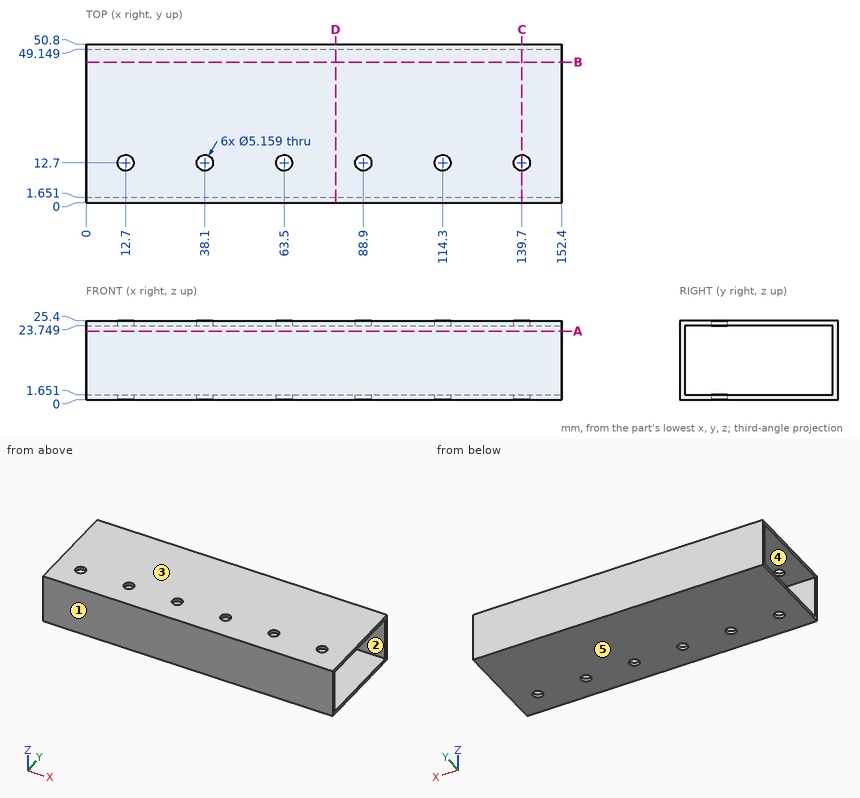
The drawing under review shows one solid part. Ordinate dimensions are in mm from its lowest x, y, z. A direction names the side the tool comes from. Coordinates: 2 decimals unless noted, no trailing zeros. Write each loop counter-clockwise with the first axis right and the second up, starting at its lowest first coordinate (ties: lowest second). Pieces come first, ordered by that corner, then holes. Notation, with made-up numbers: (6.5, 67) - (30.5, 67) arc R21 ccw to (30.5, 80) - close; hole circle Ø7 at (15, 33.25). An arc over 180 degrees is marked (long way). Use one line per item in the form item = value.
Q1. Consider section D-D (x = 80). Write out the cut boundary in (y, z).
Taken from the geometry:
outline = (0, 0) - (50.8, 0) - (50.8, 25.4) - (0, 25.4) - close; hole (1.65, 1.65) - (49.15, 1.65) - (49.15, 23.75) - (1.65, 23.75) - close
Q2. Consider section C-C (x = 139.7). Write out the cut boundary in (y, z).
Taken from the geometry:
outline = (0, 0) - (10.12, 0) - (10.12, 1.65) - (1.65, 1.65) - (1.65, 23.75) - (10.12, 23.75) - (10.12, 25.4) - (0, 25.4) - close; (15.28, 0) - (50.8, 0) - (50.8, 25.4) - (15.28, 25.4) - (15.28, 23.75) - (49.15, 23.75) - (49.15, 1.65) - (15.28, 1.65) - close
Q3. The part is to be moulded in two halves that separate along Z. For the marked faces 3, 4 and 5, say which applies: +Z half, -Z half, draft (parallel to the pull), parting line (faces both ways), or undercut.
Taken from the geometry:
face_3 = +Z half
face_4 = undercut
face_5 = -Z half
Q4. Machinability: for the marked faces 1 and 2, which of the approach directions +Z, -Z, +X, -X, +Y, -Y give a long, thin tool a straight path to every point of the face, cutting with its end or side? Answer none if there is none.
Taken from the geometry:
face_1 = +Z, -Z, +X, -X, -Y
face_2 = +X, -X
Q5. Consider section B-B (y = 45). Write out the cut boundary in (x, z).
Taken from the geometry:
outline = (0, 0) - (152.4, 0) - (152.4, 1.65) - (0, 1.65) - close; (0, 23.75) - (152.4, 23.75) - (152.4, 25.4) - (0, 25.4) - close
Q6. For probe 1 along Z at (x, y) = (99.5, 6.5); probe 2 along Y at (x, z) = (12.7, 0.9); probe 3 along Y at (x, z) = (20.5, 11.75), list the stretches that pass through material, from the lowest coordinate up.
Taken from the geometry:
probe_1 = 0 to 1.65, 23.75 to 25.4
probe_2 = 0 to 10.12, 15.28 to 50.8
probe_3 = 0 to 1.65, 49.15 to 50.8
Q7. Consider section A-A (z = 22). Write out the cut boundary in (x, y).
Taken from the geometry:
outline = (0, 0) - (152.4, 0) - (152.4, 1.65) - (0, 1.65) - close; (0, 49.15) - (152.4, 49.15) - (152.4, 50.8) - (0, 50.8) - close
